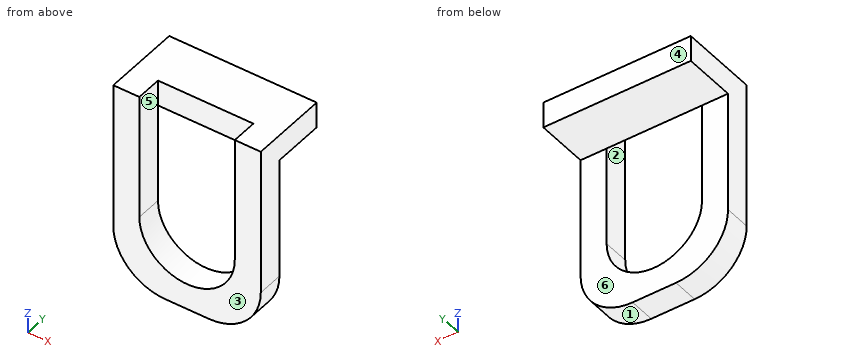
```python
from build123d import *

# Parameters (mm, degrees)
F0_W          = 53.975
F0_H          = 19.05
F1_DEPTH      = 9.525
F2_W          = 53.975
F2_H          = 9.525
F3_DEPTH      = 9.525
F3_DEPTH_BACK = 63.5
F5_DEPTH      = 9.525
F6_R          = 19.05


with BuildPart() as f1:
    # F0 (on Top) → F1 (new body)
    with BuildSketch(Plane.XY):
        with Locations((0, 9.525)):
            Rectangle(F0_W, F0_H)
    extrude(amount=F1_DEPTH)

    # F2 (on Top) → F3 (join, two sides)
    with BuildSketch(Plane.XY) as f3_sk:
        with Locations((0, -4.7625)):
            Rectangle(F2_W, F2_H)
    extrude(amount=F3_DEPTH)
    extrude(f3_sk.sketch, amount=-F3_DEPTH_BACK)

    # F4 (on face) → F5 (cut)
    with BuildSketch(Plane.XZ.offset(9.525)):
        with BuildLine():
            Line((17.4625, 9.525), (-17.4625, 9.525))
            Line((-17.4625, 9.525), (-17.4625, -36.5125))
            ThreePointArc((-17.4625, -36.5125), (0, -53.975), (17.4625, -36.5125))
            Line((17.4625, -36.5125), (17.4625, 9.525))
        make_face()
    extrude(amount=-F5_DEPTH, mode=Mode.SUBTRACT)

    # F6
    f6_edges = [f1.edges().sort_by_distance(p)[0] for p in [
        (26.9875, -4.7625, -63.5),
        (-26.9875, -4.7625, -63.5),
    ]]
    fillet(f6_edges, radius=F6_R)


solid = f1.part
```
The listing builds one solid part. Answer for the finished solid, in the listing's coordinates (mm). Face numbers are marked on the shaded views. A direction names the side the tool comes from. Round coordinates to 2 decimals unless told otherwise and drop trailing zeros. Loops run counter-clockwise (first coordinate to the right, second up) from the corner with the lowest first, then second, coordinate; pieces in that order, holes last.
Q1. Section D-D, the plane y = 3.75 is taken. Determine the outline of the cut face in (x, z) (1 decimal), then the cut area to 3 significant figures.
Q2. Section A-A, the plane z = -34.5 is taken. Determine the outline of the cut face in (x, y) (1 decimal), then the cut area to 3 significant figures.
Q3. Find the intervals of material crossed by line 1 (X direction, y = -2.75, z = -26); line 2 (Z direction, x = 22.5, y = 1) (3 decimals); line 3 (Y direction, x = 8, z = -59) (3 decimals), in increasing order.
Q4. Given pin 1 Ø7.5 at (x, z) = (1.5, 5.5) entering from -Y, flat-ended and moving along its own axis, determine where the tip first touches the part or whether it passes through.
Q5. Which of the six approach directions +Z, -Z, +X, -X, +Y, -Y give full straight-line access (tool end or side, diameter ignored) to the marked faces 4, 5 and 6?
Q6. Section B-B, the plane x = 0 is taken. Determine the outline of the cut face in (y, z) (3 decimals), then the cut area to 3 significant figures.
Q7. For a pull along X with two mould halves and no side action, classify the marked faces 1, 2 and 3 as released by +X, released by -X, zero draft, split by the parting line, or undercut.
Completed:
1. outline: (-27, 0) - (27, 0) - (27, 9.5) - (-27, 9.5) - close
1. area: 514 mm2
2. outline: (-27, -9.5) - (-17.5, -9.5) - (-17.5, 0) - (-27, 0) - close; (17.5, -9.5) - (27, -9.5) - (27, 0) - (17.5, 0) - close
2. area: 181 mm2
3. line 1: x = -26.99 to -17.46, 17.46 to 26.99
3. line 2: z = 0 to 9.525
3. line 3: y = -9.525 to 0
4. pin 1: stops at y = 0
5. face 4: +Z, -Z, +X, -X, +Y
5. face 5: +Z, -Y
5. face 6: -Z, +X, -X, +Y
6. outline: (-9.525, -63.5) - (0, -63.5) - (0, -53.975) - (-9.525, -53.975) - close; (0, 0) - (19.05, 0) - (19.05, 9.525) - (0, 9.525) - close
6. area: 272 mm2
7. face 1: released by +X
7. face 2: undercut
7. face 3: zero draft
